Geometry: see drawing. Coordinates: mm, zero at the bounding-box minimum. Give positions to 0.01 mm unless a question says otherwise; leave off trailing zeros. Order: outer loops, then holes, each group sorted by start corner. A loop starts at its lowest first (then second) coordinate and runs counter-clockwise, first axis right, second up. Notation, with made-up numbers: (17, -6) - (53, -6) arc R24 ccw to (53, 28) - close; hole circle Ø1 at (17, -31.5). An arc over 180 degrees is marked (long way). Write each question's results on one line, items separated by ' | '. Start each with the question number.
Item 1: Section B-B on y = 13. Output: boundary loops of the cut face in (x, z), and give its area (3 significant figures).
Item 2: Contact query for flat-ended pins moving along their axis: pin 1 Ø6 at (x, z) = (13, 11) entering from +Y; pin 2 Ø3.5 at (x, y) = (99, 8.5) entering from +Z; pin 3 Ø3.5 at (x, y) = (98.5, 7) entering from -Z. Output: stop coordinate, or through.
Item 3: Section C-C on x = 83. Output: boundary loops of the cut face in (y, z), and give its area (3 significant figures).
Item 4: Mould query, pull axis X, two halves, no side actions, for the marked faces 1, 2 and 3. Classes: released by +X, released by -X, zero draft, split by the parting line, or undercut.
Item 5: Section D-D on y = 4.75. Output: boundary loops of the cut face in (x, z).
Item 6: Section A-A on z = 25. Output: boundary loops of the cut face in (x, y), and give its area (3 significant figures).
Item 7: Line query: line 1 along Y through (x, z) = (17, 2); line 2 along X through (y, z) = (6.5, 6.5). Output: solid intervals per line, ascending.
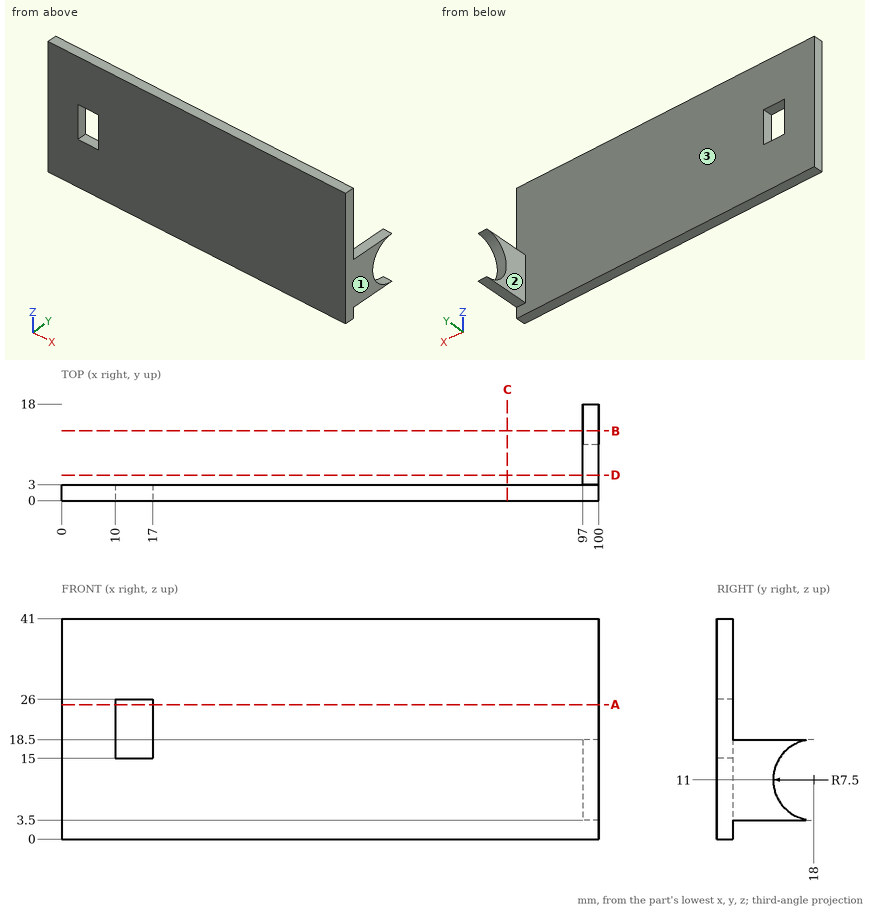
Evaluation:
1) outline: (97, 3.5) - (100, 3.5) - (100, 5.41) - (97, 5.41) - close; (97, 16.59) - (100, 16.59) - (100, 18.5) - (97, 18.5) - close | area: 11.5 mm^2
2) pin 1: stops at y = 3 | pin 2: stops at z = 18.5 | pin 3: stops at z = 3.5
3) outline: (0, 0) - (3, 0) - (3, 41) - (0, 41) - close | area: 123 mm^2
4) face 1: released by +X | face 2: released by -X | face 3: zero draft
5) outline: (97, 3.5) - (100, 3.5) - (100, 18.5) - (97, 18.5) - close
6) outline: (0, 0) - (10, 0) - (10, 3) - (0, 3) - close; (17, 0) - (100, 0) - (100, 3) - (17, 3) - close | area: 279 mm^2
7) line 1: y = 0 to 3 | line 2: x = 97 to 100
